Could you check a few things on this model? Use its own coordinates, in mm. Coordinates: 2 decimals unless noted, no trailing zeros. Order: outer loops, then holes, each group sorted by start corner. A loop starts at its lowest first (then second) coordinate and runs counter-clockwise, first axis right, second up. Notation, with made-up numbers: (-2, 46.5) -> (57, 46.5) arc R6 ccw to (57, 57.5) -> close; hole circle Ø4 at (44.5, 30). An arc over 180 degrees is marked (long way). Put each result on its own line as item: value. Start each with the question number.
Q1. If we section it at D-D (x = 17): Please give me the cut outline in (y, z).
Q2. We'd pull the mould along Z, two halves only. Please class faces 1 (the face through (0, 0.3, -23)), 2 (the face through (-11.9, 0.15, -9.13)): +Z half, -Z half, draft (parallel to the pull), parting line (faces both ways), or undercut.
Q3. Please list where these lines run through material, in increasing order: line 1 along Z through (x, y) = (1, 0.25); line 2 along X through (y, z) = (0.2, -50); line 3 along Z through (x, y) = (-8, 0.2).
Q4. Will this pin go through, and if not, where does the flat tip stop? pin 1 (24 mm diameter, centred on x = 0, z = 0, fed in from -Y).
Q5. If we section it at A-A (z = -50): Please give me the cut outline in (x, y).
Q6. If we section it at C-C (y = 0.25): Please give me the cut outline in (x, z), and give its area (3 significant figures).
Q7. If we section it at B-B (x = 0): Please give me the cut outline in (y, z), and give its area (3 significant figures).
from build123d import *

# Parameters (mm, degrees)
SKETCH1_R           = 20
SKETCH1_R_2         = 10
SKETCH1_R_3         = 25
SKETCH1_R_4         = 15
SKETCH1_W           = 17.5
SKETCH1_H           = 25
BOSS_EXTRUDE1_DEPTH = 0.3


with BuildPart() as part:
    # Sketch1 → Boss-Extrude1 (new body)
    with BuildSketch(Plane(origin=(0, 0, 0), x_dir=(1, 0, 0), z_dir=(0, 1, 0))):
        with Locations((0, 50)):
            Circle(SKETCH1_R)
        with Locations((0, 50)):
            Circle(SKETCH1_R_2, mode=Mode.SUBTRACT)
        Circle(SKETCH1_R_3)
        Circle(SKETCH1_R_4, mode=Mode.SUBTRACT)
        with Locations((0, 27.5)):
            Rectangle(SKETCH1_W, SKETCH1_H)
    extrude(amount=BOSS_EXTRUDE1_DEPTH)


solid = part.part
The answers:
1. outline: (0, -60.54) -> (0.3, -60.54) -> (0.3, -39.46) -> (0, -39.46) -> close; (0, -18.33) -> (0.3, -18.33) -> (0.3, 18.33) -> (0, 18.33) -> close
2. face 1: draft
2. face 2: undercut
3. line 1: -69.97 to -59.95, -40.05 to -14.97, 14.97 to 24.98
3. line 2: -20 to -10, 10 to 20
3. line 3: -68.33 to -56, -44 to -12.69, 12.69 to 23.69
4. pin 1: through
5. outline: (-20, 0) -> (-10, 0) -> (-10, 0.3) -> (-20, 0.3) -> close; (10, 0) -> (20, 0) -> (20, 0.3) -> (10, 0.3) -> close
6. outline: (-8.75, -32.02) arc R20 ccw (long way) to (8.75, -32.02) -> (8.75, -23.42) arc R25 ccw (long way) to (-8.75, -23.42) -> close; hole circle Ø30 at (0, 0); hole circle Ø20 at (0, -50)
6. area: 2,310 mm^2
7. outline: (0, -70) -> (0.3, -70) -> (0.3, -60) -> (0, -60) -> close; (0, -40) -> (0.3, -40) -> (0.3, -15) -> (0, -15) -> close; (0, 15) -> (0.3, 15) -> (0.3, 25) -> (0, 25) -> close
7. area: 13.5 mm^2
